```python
from build123d import *

# Parameters (mm, degrees)
BASE_FLANGE1_DEPTH         = 3.175
F_5_2_5_2_DIAMETER_HOLE1_D = 5.2


# Sheet-metal steps are written as plain solids
with BuildPart() as part:
    # Sketch11 → Base-Flange1 (new body)
    with BuildSketch(Plane(origin=(0, 0, -167.271453779), x_dir=(-1, 0, 0), z_dir=(0, 0, -1))):
        with BuildLine():
            Line((395.316058397, 315.309736729), (425.316058397, 315.309736729))
            Line((425.316058397, 315.309736729), (425.316058397, 285.309736729))
            ThreePointArc((425.316058397, 285.309736729), (435.316058397, 275.309736729), (445.316058397, 285.309736729))
            Line((445.316058397, 285.309736729), (445.316058397, 332.809736729))
            ThreePointArc((445.316058397, 332.809736729), (444.58382535, 334.577503682), (442.816058397, 335.309736729))
            Line((442.816058397, 335.309736729), (395.316058397, 335.309736729))
            ThreePointArc((395.316058397, 335.309736729), (385.316058397, 325.309736729), (395.316058397, 315.309736729))
        make_face()
    extrude(amount=-BASE_FLANGE1_DEPTH)

    # Ø5.2 (5.2) Diameter Hole1 (through all)
    with Locations(Plane(origin=(0, 0, -167.271453779), x_dir=(-1, 0, 0), z_dir=(0, 0, -1))):
        with Locations((435.316058397, 285.309736729), (395.316058397, 325.309736729), (415.316058397, 325.309736729), (435.316058397, 305.336856842)):
            Hole(F_5_2_5_2_DIAMETER_HOLE1_D / 2)


solid = part.part
```
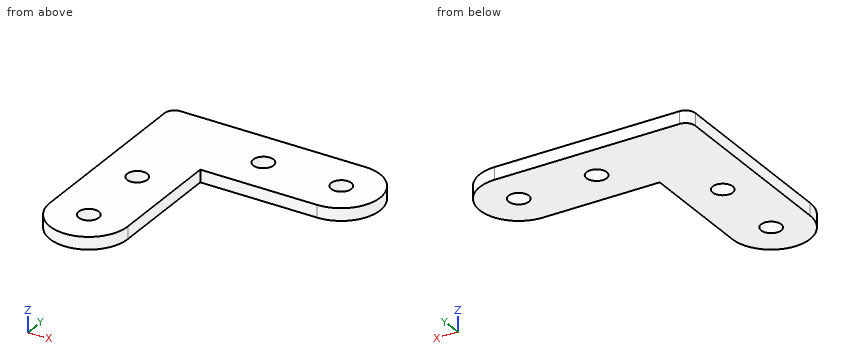
Geometry: final body of the model. Coordinates: model frame, mm. Round coordinates to 2 decimals unless told otherwise and drop trailing zeros. Loops run counter-clockwise (first coordinate to the right, second up) from the corner with the lowest first, then second, coordinate; pieces in that order, holes last.
Item 1: Section D-D, the plane y = 324. Output: boundary loops of the cut face in (x, z), plus the area to 3 significant figures.
Checked values:
outline: (-445.32, -167.27) - (-417.56, -167.27) - (-417.56, -164.1) - (-445.32, -164.1) - close; (-413.07, -167.27) - (-397.56, -167.27) - (-397.56, -164.1) - (-413.07, -164.1) - close; (-393.07, -167.27) - (-385.4, -167.27) - (-385.4, -164.1) - (-393.07, -164.1) - close
area: 162 mm2
Item 2: Contact query for flat-ended pins moving along their axis: P1, Ø3, axis at x = -415.32, y = 325.31, coming from the -Z side; P2, Ø1.6, axis at y = 293.5, z = -166, coming from the +X side; P3, Ø1.5, axis at y = 321.5, z = -164.5, coming from the +X side. Output: stop coordinate, or through.
Checked values:
P1: passes through
P2: stops at x = -425.32
P3: stops at x = -385.8
Item 3: Section A-A, the plane y = 284.5. Output: boundary loops of the cut face in (x, z).
Checked values:
outline: (-445.28, -167.27) - (-437.79, -167.27) - (-437.79, -164.1) - (-445.28, -164.1) - close; (-432.85, -167.27) - (-425.35, -167.27) - (-425.35, -164.1) - (-432.85, -164.1) - close
Item 4: Section C-C, the plane z = -165.3. Output: boundary loops of the cut face in (x, y), plus the area to 3 significant figures.
Checked values:
outline: (-445.32, 285.31) arc R10 ccw to (-425.32, 285.31) - (-425.32, 315.31) - (-395.32, 315.31) arc R10 ccw to (-395.32, 335.31) - (-442.82, 335.31) arc R2.5 ccw to (-445.32, 332.81) - close; hole circle Ø5.2 at (-435.32, 285.31); hole circle Ø5.2 at (-435.32, 305.34); hole circle Ø5.2 at (-415.32, 325.31); hole circle Ø5.2 at (-395.32, 325.31)
area: 1,830 mm2
Item 5: Section B-B, the plane x = -413.5. Output: boundary loops of the cut face in (y, z).
Checked values:
outline: (315.31, -167.27) - (323.45, -167.27) - (323.45, -164.1) - (315.31, -164.1) - close; (327.17, -167.27) - (335.31, -167.27) - (335.31, -164.1) - (327.17, -164.1) - close
Item 6: Line query: L1, parallel to X at y = 307, z = -164.2; L2, parallel to Y at x = -437.5, z = -167.05; L3, parallel to Y at x = -400.5, z = -164.7. Output: solid intervals per line, ascending.
Checked values:
L1: x = -445.32 to -437.31, -433.32 to -425.32
L2: y = 275.55 to 283.9, 286.72 to 303.93, 306.75 to 335.31
L3: y = 315.31 to 335.31
